Check sheet for the modelled part. Datum: model origin and axes. Units: mm. A direction names the side the tool comes from. Round coordinates to 2 decimals unless told otherwise and drop trailing zeros.
Item 1: Release check for a two-part mould opening along Y. For faces 1 (the flat face through (-5, -57, 0)), 2 (the cylindrical face through (-49.731, 51.926, -0.479)) record: pulls with the +Y half, pulls with the -Y half, needs draft (parallel to the pull), parting line crosses it, or undercut.
Item 2: Set-up check for faces 3 (the flat face through (52.3, 53.1, 1)), 4 (the flat face through (-49, 50, -2)), 5 (the flat face through (1, 1, 0)): record each of +Z, -Z, +X, -X, +Y, -Y from which the full face is reachable in a straight line by a thin tool's end or side.
Item 3: Depth check by flat-ended pin: pin 1 (3 mm diameter, centred on x = -51.4, y = -51.4, fed in from -Z); pin 2 (2 mm diameter, centred on x = -53, y = 52.5, fed in from +Z); pin 3 (0.8 mm diameter, centred on y = 6, z = -1, fed in from +X); pin 4 (1.2 mm diameter, centred on y = 12, z = -1, fed in from -X). Enter the tip coordinate at first touch or a pass-through.
Item 4: Material ranges on line 1 along Y through (x, z) = (51.4, 2.5); line 2 along Y through (x, z) = (-52.5, 1.6); line 3 along Y through (x, z) = (51.4, -0.85), recorded low to high.
from build123d import *

# Parameters (mm, degrees)
ESBO_O1_W                 = 120
ESBO_O1_H                 = 120
RESSALTO_EXTRUS_O1_DEPTH  = 3
ESBO_O2_W                 = 112.8
ESBO_O2_H                 = 112.8
RESSALTO_EXTRUS_O2_DEPTH  = 2
ESBO_O3_W                 = 108.8
ESBO_O3_H                 = 108.8
CORTE_EXTRUS_O1_DEPTH     = 2
ESBO_O5_R                 = 5
RESSALTO_EXTRUS_O3_DEPTH  = 2
ESPELHAR2_COPY_1_SKETCH_R = 5
ESPELHAR2_COPY_1_DEPTH    = 2
CHANFRO1_SIZE             = 0.5
FILETE1_R                 = 2
ESBO_O6_R                 = 3.6
CORTE_EXTRUS_O2_DEPTH     = 2
ESBO_O7_R                 = 1.75
CORTE_EXTRUS_O3_DEPTH     = 85.905830189
ESPELHAR4_COPY_1_SKETCH_R = 3.6
ESPELHAR4_COPY_1_DEPTH    = 2
ESPELHAR4_COPY_2_SKETCH_R = 1.75
ESPELHAR4_COPY_2_DEPTH    = 85.905830189
FILETE2_R                 = 0.5


with BuildPart() as part:
    # Esboço1 → Ressalto-extrusão1 (new body)
    with BuildSketch(Plane.XY):
        Rectangle(ESBO_O1_W, ESBO_O1_H)
    extrude(amount=RESSALTO_EXTRUS_O1_DEPTH)

    # Esboço2 → Ressalto-extrusão2 (add)
    with BuildSketch(Plane(origin=(0, 0, 0), x_dir=(-1, 0, 0), z_dir=(0, 0, -1))):
        Rectangle(ESBO_O2_W, ESBO_O2_H)
    extrude(amount=RESSALTO_EXTRUS_O2_DEPTH)

    # Esboço3 → Corte-extrusão1 (cut)
    with BuildSketch(Plane(origin=(0, 0, -2), x_dir=(-1, 0, 0), z_dir=(0, 0, -1))):
        Rectangle(ESBO_O3_W, ESBO_O3_H)
    extrude(amount=-CORTE_EXTRUS_O1_DEPTH, mode=Mode.SUBTRACT)

    # Esboço5 → Ressalto-extrusão3 (add)
    with BuildSketch(Plane(origin=(0, 0, 0), x_dir=(-1, 0, 0), z_dir=(0, 0, -1))):
        with Locations((51.4, 51.4)):
            Circle(ESBO_O5_R)
    ressalto_extrus_o3 = extrude(amount=RESSALTO_EXTRUS_O3_DEPTH)

    # Espelhar1: Ressalto-extrusão3 across plane
    add(ressalto_extrus_o3.mirror(Plane(origin=(0, 0, 0), x_dir=(0, 0, 1), z_dir=(1, 0, 0))))

    # Espelhar2: Ressalto-extrusão3 across plane
    add(ressalto_extrus_o3.mirror(Plane.ZX))

    # Espelhar2 copy 1 sketch → Espelhar2 copy 1 (add)
    with BuildSketch(Plane(origin=(0, 0, 0), x_dir=(1, 0, 0), z_dir=(0, 0, -1))):
        with Locations((51.4, 51.4)):
            Circle(ESPELHAR2_COPY_1_SKETCH_R)
    extrude(amount=ESPELHAR2_COPY_1_DEPTH)

    # Chanfro1
    chanfro1_edges = [part.edges().sort_by_distance(p)[0] for p in [
        (0, 56.4, -2),
        (56.4, 0, -2),
        (0, -56.4, -2),
        (-56.4, 0, -2),
    ]]
    chamfer(chanfro1_edges, length=CHANFRO1_SIZE)

    # Filete1
    filete1_edges = [part.edges().sort_by_distance(p)[0] for p in [
        (0, -54.4, 0),
        (47.864466094, -47.864466094, 0),
        (54.4, 0, 0),
        (47.864466094, 47.864466094, 0),
        (0, 54.4, 0),
        (-47.864466094, 47.864466094, 0),
        (-54.4, 0, 0),
        (-47.864466094, -47.864466094, 0),
    ]]
    fillet(filete1_edges, radius=FILETE1_R - 0.0001)  # a hair under: the kernel refuses the full size

    # Esboço6 → Corte-extrusão2 (cut)
    with BuildSketch(Plane.XY.offset(3)):
        with Locations((-51.4, 51.4)):
            Circle(ESBO_O6_R)
    corte_extrus_o2 = extrude(amount=-CORTE_EXTRUS_O2_DEPTH, mode=Mode.SUBTRACT)

    # Esboço7 → Corte-extrusão3 (cut, through all)
    with BuildSketch(Plane.XY.offset(1)):
        with Locations((-51.4, 51.4)):
            Circle(ESBO_O7_R)
    corte_extrus_o3 = extrude(amount=-CORTE_EXTRUS_O3_DEPTH, mode=Mode.SUBTRACT)

    # Espelhar3: Corte-extrusão2, Corte-extrusão3 across plane
    add(corte_extrus_o2.mirror(Plane(origin=(0, 0, 0), x_dir=(0, 0, 1), z_dir=(1, 0, 0))), mode=Mode.SUBTRACT)
    add(corte_extrus_o3.mirror(Plane(origin=(0, 0, 0), x_dir=(0, 0, 1), z_dir=(1, 0, 0))), mode=Mode.SUBTRACT)

    # Espelhar4: Corte-extrusão2, Corte-extrusão3 across plane
    add(corte_extrus_o2.mirror(Plane.ZX), mode=Mode.SUBTRACT)
    add(corte_extrus_o3.mirror(Plane.ZX), mode=Mode.SUBTRACT)

    # Espelhar4 copy 1 sketch → Espelhar4 copy 1 (cut)
    with BuildSketch(Plane(origin=(0, 0, 3), x_dir=(-1, 0, 0), z_dir=(0, 0, 1))):
        with Locations((-51.4, 51.4)):
            Circle(ESPELHAR4_COPY_1_SKETCH_R)
    extrude(amount=-ESPELHAR4_COPY_1_DEPTH, mode=Mode.SUBTRACT)

    # Espelhar4 copy 2 sketch → Espelhar4 copy 2 (cut, through all)
    with BuildSketch(Plane(origin=(0, 0, 1), x_dir=(-1, 0, 0), z_dir=(0, 0, 1))):
        with Locations((-51.4, 51.4)):
            Circle(ESPELHAR4_COPY_2_SKETCH_R)
    extrude(amount=-ESPELHAR4_COPY_2_DEPTH, mode=Mode.SUBTRACT)

    # Filete2
    filete2_edges = [part.edges().sort_by_distance(p)[0] for p in [
        (-60, 0, 3),
        (0, -60, 3),
        (60, 0, 3),
        (0, -60, 0),
        (-60, 0, 0),
        (0, 60, 0),
        (60, 0, 0),
        (60, -60, 1.5),
        (-60, -60, 1.5),
        (-60, 60, 1.5),
        (60, 60, 1.5),
        (0, 60, 3),
    ]]
    fillet(filete2_edges, radius=FILETE2_R)


solid = part.part
Values found:
1. face 1: needs draft
1. face 2: undercut
2. face 3: +Z
2. face 4: -Z, +X, -X, +Y, -Y
2. face 5: -Z
3. pin 1: passes through
3. pin 2: stops at z = 1
3. pin 3: stops at x = 56.4
3. pin 4: stops at x = -56.4
4. line 1: y = -60 to -55, -47.8 to 47.8, 55 to 60
4. line 2: y = -60 to -54.83, -47.97 to 47.97, 54.83 to 60
4. line 3: y = -56.4 to -53.15, -49.65 to -46.04, 46.04 to 49.65, 53.15 to 56.4
